from build123d import *

# Parameters (mm, degrees)
SKETCH3_R               = 1.27
CUT_EXTRUDE1_DEPTH      = 5.572
CUT_EXTRUDE1_DEPTH_BACK = 5.572
SKETCH4_R               = 1.27
CUT_EXTRUDE2_DEPTH      = 5.5720001
CUT_EXTRUDE2_DEPTH_BACK = 5.5720001


with BuildPart() as part:
    # Sketch2 → Revolve1 (revolve)
    with BuildSketch(Plane(origin=(0, 0, 0), x_dir=(1, 0, 0), z_dir=(0, 1, 0))):
        Polygon((0, 0), (0, -19.05), (4.572, -19.05), (4.572, -10.5791), (4.064, -10.5791), (4.064, -8.4709), (4.572, -8.4709), (4.572, 0), align=None)
    revolve(axis=Axis((0, 0, 0), (0, 0, 1)))

    # Sketch3 → Cut-Extrude1 (cut, two sides)
    with BuildSketch(Plane(origin=(0, 0, 0), x_dir=(1, 0, 0), z_dir=(0, 1, 0))) as cut_extrude1_sk:
        with Locations((0, -12.446)):
            Circle(SKETCH3_R)
    extrude(amount=CUT_EXTRUDE1_DEPTH, mode=Mode.SUBTRACT)
    extrude(cut_extrude1_sk.sketch, amount=-CUT_EXTRUDE1_DEPTH_BACK, mode=Mode.SUBTRACT)

    # Sketch4 → Cut-Extrude2 (cut, two sides)
    with BuildSketch(Plane(origin=(0, 0, 0), x_dir=(0, 0, -1), z_dir=(1, 0, 0))) as cut_extrude2_sk:
        with Locations((-2.54, 0)):
            Circle(SKETCH4_R)
        with Locations((-16.51, 0)):
            Circle(SKETCH4_R)
    extrude(amount=CUT_EXTRUDE2_DEPTH, mode=Mode.SUBTRACT)
    extrude(cut_extrude2_sk.sketch, amount=-CUT_EXTRUDE2_DEPTH_BACK, mode=Mode.SUBTRACT)


solid = part.part
Part model, mm, in its own coordinate system. A direction names the side the tool comes from. Round coordinates to 2 decimals unless told otherwise and drop trailing zeros. Write each loop counter-clockwise with the first axis right and the second up, starting at its lowest first coordinate (ties: lowest second). Pieces come first, ordered by that corner, then holes. Notation, with made-up numbers: M 77.25,81 L 81.25,81 A23 ccw 81.25,97 Z; hole C 25.25,-37.5 d10. An arc over 180 degrees is marked long. Return JSON: item names as keys, results as strings. Group by question number.
(1) Two-plate mould, pull along Z, no slides. Class faces 1 (the face through (0, 0, 0)), 2 (the face through (0, 0, 19.05)), 3 (the face through (-3, -3, 10.579)): +Z half, -Z half, draft (parallel to the pull), parting line (faces both ways), or undercut.
(2) Saw through at A-A on x = 0.25. Write the cut outline in (y, z).
(3) Which spindle directions (+Z, -Z, +X, -X, +Y, -Y) get a long thin tool onto all of the face, cutting with end or side? Do faces 4 (the face through (4.223, -1.751, 4.176)), 5 (the face through (3, -3, 8.471)). Say none if no direction does.
(4) Saw through at D-D on x = -2. Write the cut outline in (y, z), then the cut area to 3 significant figures.
(5) Saw through at C-C on z = 11.5. Write the cut outline in (x, y), then the cut area to 3 significant figures.
(6) Pin check, flat tips, straight feed: pin 1 Ø1.5 at (y, z) = (0, 16.51) entering from +X; pin 2 Ø3 at (x, z) = (-2, 15.5) entering from +Y; pin 3 Ø3 at (y, z) = (3.5, 4) entering from +X; pin 4 Ø3 at (x, z) = (2.5, 10) entering from -Y. Stop position of each tip, or through.
(7) Saw through at B-B on y = -2. Write the cut outline in (x, z).
(8) Drill centre lines: probe 1 along Z at (x, y) = (-3.25, 0); probe 2 along Y at (x, z) = (2.1, 16.51); probe 3 along Z at (x, y) = (3.5, 2.25). Where is each one in solid material? Low to high.
Returned:
{
 "1": {"face 1": "-Z half", "face 2": "+Z half", "face 3": "undercut"},
 "2": {"outline": "M -4.57,0 L 4.57,0 L 4.57,8.47 L 4.06,8.47 L 4.06,10.58 L 4.57,10.58 L 4.57,11.2 L -4.57,11.2 L -4.57,10.58 L -4.06,10.58 L -4.06,8.47 L -4.57,8.47 Z; M -4.57,13.69 L 4.57,13.69 L 4.57,19.05 L -4.57,19.05 Z; hole C 0,2.54 d2.54; hole C 0,16.51 d2.54"},
 "3": {"face 4": "+Z, -Z", "face 5": "none"},
 "4": {"outline": "M -4.11,0 L 4.11,0 L 4.11,8.47 L 3.54,8.47 L 3.54,10.58 L 4.11,10.58 L 4.11,19.05 L -4.11,19.05 L -4.11,10.58 L -3.54,10.58 L -3.54,8.47 L -4.11,8.47 Z; hole C 0,2.54 d2.54; hole C 0,16.51 d2.54", "area": "144 mm²"},
 "5": {"outline": "M -0.85,-4.49 L -0.85,4.49 A4.57 ccw Z; M 0.85,-4.49 A4.57 ccw 0.85,4.49 Z", "area": "50.3 mm²"},
 "6": {"pin 1": "through", "pin 2": "y = 4.54", "pin 3": "x = 4.11", "pin 4": "y = -4.43"},
 "7": {"outline": "M -4.11,0 L 4.11,0 L 4.11,8.47 L 3.54,8.47 L 3.54,10.58 L 4.11,10.58 L 4.11,19.05 L -4.11,19.05 L -4.11,10.58 L -3.54,10.58 L -3.54,8.47 L -4.11,8.47 Z; hole C 0,12.45 d2.54"},
 "8": {"probe 1": "0 to 1.27, 3.81 to 15.24, 17.78 to 19.05", "probe 2": "-4.06 to -1.27, 1.27 to 4.06", "probe 3": "0 to 8.47, 10.58 to 19.05"}
}
